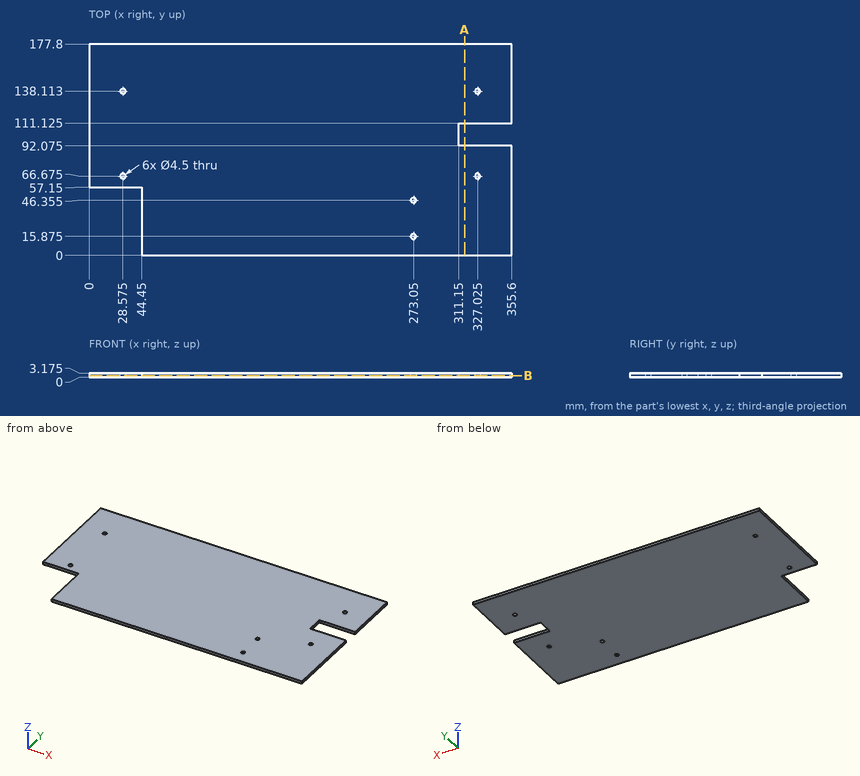
Part print with two shaded views. Sizes in mm from the minimum x, y, z corner. Round coordinates to 2 decimals unless told otherwise and drop trailing zeros. Write each loop counter-clockwise with the first axis right and the second up, starting at its lowest first coordinate (ties: lowest second). Pieces come first, ordered by that corner, then holes. Notation, with made-up numbers: M -36,3.25 L -4,3.25 A33 ccw -4,42.25 Z; hole C -22.75,1 d8. An arc over 180 degrees is marked long. Use CSV: the item, a comma, the result in double quotes.
1. Wall check: probe 1 along Y at (x, z) = (273.05, 1.3) (1 decimal); probe 2 along X at (y, z) = (137, 1.85); probe 3 along X at (y, z) = (137.5, 0.65). Give the ranges that are in metal, low to high. Write a range as from..to.
Reply:
probe 1,"y = 0..13.6, 18.1..44.1, 48.6..177.8"
probe 2,"x = 0..26.62, 30.53..325.07, 328.98..355.6"
probe 3,"x = 0..26.41, 30.74..324.86, 329.19..355.6"
2. Flat gauge pin, fed straight in: pin 1 (1 mm diameter, centred on y = 98.5, z = 1.5, fed in from +X). Where does the tip first touch, or does it go through?
Reply:
pin 1,"stops at x = 311.15"
3. Saw through at A-A (x = 316). Give the cut face in (y, z) (1 decimal), plus the area to 3 significant figures.
Reply:
outline,"M 0,0 L 92.1,0 L 92.1,3.2 L 0,3.2 Z; M 111.1,0 L 177.8,0 L 177.8,3.2 L 111.1,3.2 Z"
area,"504 mm²"
4. Saw through at B-B (z = 1.25). State how many separate pieces and enclosed holes the cut face has, plus the area to 3 significant figures.
Reply:
separate pieces,"1"
enclosed holes,"6"
area,"59,700 mm²"
